Read the model definition and answer for the solid it produces. Units are mm, in the model's axes. Face numbers are marked on the shaded views. A direction names the side the tool comes from. Coordinates: 2 decimals unless noted, no trailing zeros. Loops run counter-clockwise (first coordinate to the right, second up) from the corner with the lowest first, then second, coordinate; pieces in that order, holes last. Notation, with made-up numbers: (-27.5, -12.5) -> (-20.5, -12.5) arc R19 cw to (-20.5, 17.5) -> close; hole circle Ø4 at (47.5, 43.5). An arc over 180 degrees is marked (long way). Answer as CSV lines item,"result".
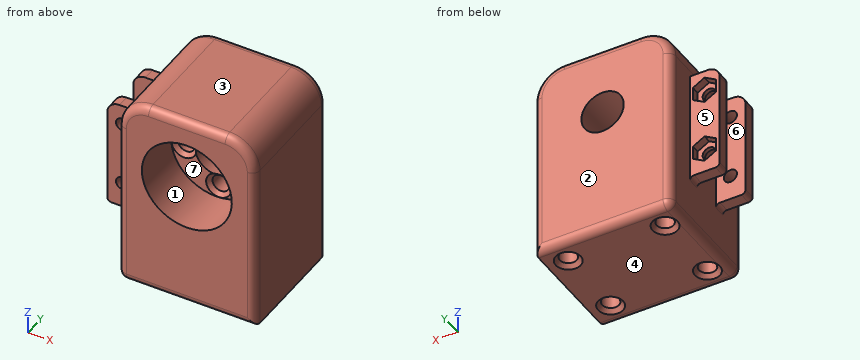
```python
from build123d import *

# Parameters (mm, degrees)
SKETCH1_W           = 34
SKETCH1_H           = 30
BOSS_EXTRUDE1_DEPTH = 49
SKETCH2_R           = 2.1
CUT_EXTRUDE1_DEPTH  = 6
SKETCH5_R           = 11.15
CUT_EXTRUDE2_DEPTH  = 12.5
SKETCH6_R           = 5.25
CUT_EXTRUDE3_DEPTH  = 17.5
SKETCH7_R           = 2.1
CUT_EXTRUDE4_DEPTH  = 6
CHAMFER1_SIZE       = 1
CHAMFER2_SIZE       = 1
FILLET1_R           = 7.5
FILLET2_R           = 2
BOSS_EXTRUDE2_START = 4
SKETCH9_W           = 7.353949633
SKETCH9_H           = 27.286831646
SKETCH9_R           = 1.625
BOSS_EXTRUDE2_DEPTH = 3
FILLET3_R           = 3
FILLET4_R           = 1
CUT_EXTRUDE6_DEPTH  = 2


with BuildPart() as part:
    # Sketch1 → Boss-Extrude1 (new body)
    with BuildSketch(Plane.XY):
        Rectangle(SKETCH1_W, SKETCH1_H)
    extrude(amount=BOSS_EXTRUDE1_DEPTH)

    # Sketch2 → Cut-Extrude1 (cut)
    with BuildSketch(Plane(origin=(0, 0, 0), x_dir=(-1, 0, 0), z_dir=(0, 0, -1))):
        with Locations((12, -9)):
            Circle(SKETCH2_R)
        with Locations((12, 9)):
            Circle(SKETCH2_R)
        with Locations((-12, -9)):
            Circle(SKETCH2_R)
        with Locations((-12, 9)):
            Circle(SKETCH2_R)
    extrude(amount=-CUT_EXTRUDE1_DEPTH, mode=Mode.SUBTRACT)

    # Sketch5 → Cut-Extrude2 (cut)
    with BuildSketch(Plane.XZ.offset(15)):
        with Locations(Location((0, 31.713602896, 0), (0, 0, 270))):
            Circle(SKETCH5_R)
    extrude(amount=-CUT_EXTRUDE2_DEPTH, mode=Mode.SUBTRACT)

    # Sketch6 → Cut-Extrude3 (cut)
    with BuildSketch(Plane(origin=(0, 15, 0), x_dir=(1, 0, 0), z_dir=(0, 1, 0))):
        with Locations(Location((0, -31.713602896, 0), (0, 0, 270))):
            Circle(SKETCH6_R)
    extrude(amount=-CUT_EXTRUDE3_DEPTH, mode=Mode.SUBTRACT)

    # Sketch7 → Cut-Extrude4 (cut)
    with BuildSketch(Plane.XZ.offset(2.5)):
        with Locations(Location((-7.978464084, 31.126993267, 0), (0, 0, 270))):
            Circle(SKETCH7_R)
        with Locations(Location((-0.586609629, 39.692066981, 0), (0, 0, 270))):
            Circle(SKETCH7_R)
        with Locations(Location((7.978464084, 31.126993267, 0), (0, 0, 270))):
            Circle(SKETCH7_R)
        with Locations(Location((0.586609629, 23.735138812, 0), (0, 0, 270))):
            Circle(SKETCH7_R)
    extrude(amount=-CUT_EXTRUDE4_DEPTH, mode=Mode.SUBTRACT)

    # Chamfer1
    # the kernel refuses this chamfer: 1 mm, written as the material it takes off along each edge
    with BuildSketch(Plane(origin=(-7.978464084, -2.5, 31.126993267), x_dir=(0, 0, -1), z_dir=(-1, 0, 0))) as chamfer1_piece_1:
        Polygon((2.1 + CHAMFER1_SIZE, 0), (2.1, -CHAMFER1_SIZE), (2.1, 0), align=None)
    revolve(axis=Axis((-7.978464084, -2.5, 31.126993267), (0, -1, 0)), mode=Mode.SUBTRACT)
    with BuildSketch(Plane(origin=(-0.586609629, -2.5, 39.692066981), x_dir=(0, 0, -1), z_dir=(-1, 0, 0))) as chamfer1_piece_2:
        Polygon((2.1 + CHAMFER1_SIZE, 0), (2.1, -CHAMFER1_SIZE), (2.1, 0), align=None)
    revolve(axis=Axis((-0.586609629, -2.5, 39.692066981), (0, -1, 0)), mode=Mode.SUBTRACT)
    with BuildSketch(Plane(origin=(7.978464084, -2.5, 31.126993267), x_dir=(0, 0, -1), z_dir=(-1, 0, 0))) as chamfer1_piece_3:
        Polygon((2.1 + CHAMFER1_SIZE, 0), (2.1, -CHAMFER1_SIZE), (2.1, 0), align=None)
    revolve(axis=Axis((7.978464084, -2.5, 31.126993267), (0, -1, 0)), mode=Mode.SUBTRACT)
    with BuildSketch(Plane(origin=(0.586609629, -2.5, 23.735138812), x_dir=(0, 0, -1), z_dir=(-1, 0, 0))) as chamfer1_piece_4:
        Polygon((2.1 + CHAMFER1_SIZE, 0), (2.1, -CHAMFER1_SIZE), (2.1, 0), align=None)
    revolve(axis=Axis((0.586609629, -2.5, 23.735138812), (0, -1, 0)), mode=Mode.SUBTRACT)

    # Chamfer2
    chamfer2_edges = [part.edges().sort_by_distance(p)[0] for p in [
        (-9.9, 9, 0),
        (14.1, -9, 0),
        (14.1, 9, 0),
        (-9.9, -9, 0),
    ]]
    chamfer(chamfer2_edges, length=CHAMFER2_SIZE)

    # Fillet1
    fillet1_edges = [part.edges().sort_by_distance(p)[0] for p in [
        (-17, 0, 49),
        (17, 0, 49),
    ]]
    fillet(fillet1_edges, radius=FILLET1_R)

    # Fillet2
    # the kernel refuses this fillet: 2 mm, written as the material it takes off along each edge
    with BuildSketch(Plane(origin=(-15, -13, 2), x_dir=(0, 0, -1), z_dir=(0, -1, 0))) as fillet2_piece_1_section:
        Polygon((0, 0), (FILLET2_R, 0), (FILLET2_R, -FILLET2_R), (0, -FILLET2_R), align=None)
    fillet2_piece_1 = extrude(amount=FILLET2_R, mode=Mode.PRIVATE)
    fillet2_piece_1 = fillet2_piece_1 - Plane(origin=(-15, -13, 2), x_dir=(0.7071067811865475, 0, 0.7071067811865475), z_dir=(0, -1, 0)) * Sphere(FILLET2_R, mode=Mode.PRIVATE)
    add(fillet2_piece_1, mode=Mode.SUBTRACT)
    with BuildSketch(Plane(origin=(-15, 13, 2), x_dir=(0, 0, -1), z_dir=(0, 1, 0))) as fillet2_piece_2_section:
        Polygon((0, 0), (FILLET2_R, 0), (FILLET2_R, FILLET2_R), (0, FILLET2_R), align=None)
    fillet2_piece_2 = extrude(amount=FILLET2_R, mode=Mode.PRIVATE)
    fillet2_piece_2 = fillet2_piece_2 - Plane(origin=(-15, 13, 2), x_dir=(0.7071067811865475, 0, 0.7071067811865475), z_dir=(0, 1, 0)) * Sphere(FILLET2_R, mode=Mode.PRIVATE)
    add(fillet2_piece_2, mode=Mode.SUBTRACT)
    with BuildSketch(Plane(origin=(9.5, 15, 41.5), x_dir=(1, 0, 0), z_dir=(0, 0, -1))) as fillet2_piece_3:
        with BuildLine():
            CenterArc((7.5 - FILLET2_R, FILLET2_R), FILLET2_R, 270, 90)
            Line((7.5 - FILLET2_R, 0), (7.5, 0))
            Line((7.5, 0), (7.5, FILLET2_R))
        make_face()
    revolve(axis=Axis((9.5, 15, 41.5), (0, -1, 0)), revolution_arc=90, mode=Mode.SUBTRACT)
    with BuildSketch(Plane(origin=(17, -15, -5), x_dir=(-1, 0, 0), z_dir=(0, 0, 1)), Plane(origin=(17, 15, -5), x_dir=(0, -1, 0), z_dir=(0, 0, 1))) as fillet2_piece_4:
        with BuildLine():
            CenterArc((FILLET2_R, -FILLET2_R), FILLET2_R, 90, 90)
            Line((0, -FILLET2_R), (0, 0))
            Line((0, 0), (FILLET2_R, 0))
        make_face()
    extrude(amount=46.5, mode=Mode.SUBTRACT)
    with BuildSketch(Plane(origin=(-17, -15, 2), x_dir=(1, 0, 0), z_dir=(0, 0, 1)), Plane(origin=(-17, 15, 2), x_dir=(0, -1, 0), z_dir=(0, 0, 1))) as fillet2_piece_5:
        with BuildLine():
            CenterArc((FILLET2_R, FILLET2_R), FILLET2_R, 180, 90)
            Line((0, FILLET2_R), (0, 0))
            Line((0, 0), (FILLET2_R, 0))
        make_face()
    extrude(amount=39.5, mode=Mode.SUBTRACT)
    with BuildSketch(Plane(origin=(-9.5, -15, 41.5), x_dir=(-1, 0, 0), z_dir=(0, 0, -1))) as fillet2_piece_6:
        with BuildLine():
            CenterArc((7.5 - FILLET2_R, FILLET2_R), FILLET2_R, 270, 90)
            Line((7.5, FILLET2_R), (7.5, 0))
            Line((7.5, 0), (7.5 - FILLET2_R, 0))
        make_face()
    revolve(axis=Axis((-9.5, -15, 41.5), (0, 1, 0)), revolution_arc=90, mode=Mode.SUBTRACT)
    with BuildSketch(Plane(origin=(9.5, -15, 41.5), x_dir=(1, 0, 0), z_dir=(0, 0, -1))) as fillet2_piece_7:
        with BuildLine():
            CenterArc((7.5 - FILLET2_R, -FILLET2_R), FILLET2_R, 0, 90)
            Line((7.5, -FILLET2_R), (7.5, 0))
            Line((7.5, 0), (7.5 - FILLET2_R, 0))
        make_face()
    revolve(axis=Axis((9.5, -15, 41.5), (0, -1, 0)), revolution_arc=90, mode=Mode.SUBTRACT)
    with BuildSketch(Plane(origin=(22, -15, 0), x_dir=(0, 0, 1), z_dir=(-1, 0, 0))) as fillet2_piece_8:
        with BuildLine():
            CenterArc((FILLET2_R, FILLET2_R), FILLET2_R, 180, 90)
            Line((0, FILLET2_R), (0, 0))
            Line((0, 0), (FILLET2_R, 0))
        make_face()
    extrude(amount=37, mode=Mode.SUBTRACT)
    with BuildSketch(Plane(origin=(-17, -13, 0), x_dir=(1, 0, 0), z_dir=(0, 1, 0))) as fillet2_piece_9:
        with BuildLine():
            CenterArc((FILLET2_R, -FILLET2_R), FILLET2_R, 90, 90)
            Line((0, -FILLET2_R), (0, 0))
            Line((0, 0), (FILLET2_R, 0))
        make_face()
    extrude(amount=26, mode=Mode.SUBTRACT)
    with BuildSketch(Plane(origin=(-15, 15, 0), x_dir=(0, -1, 0), z_dir=(1, 0, 0))) as fillet2_piece_10:
        with BuildLine():
            CenterArc((FILLET2_R, -FILLET2_R), FILLET2_R, 90, 90)
            Line((0, -FILLET2_R), (0, 0))
            Line((0, 0), (FILLET2_R, 0))
        make_face()
    extrude(amount=37, mode=Mode.SUBTRACT)
    with BuildSketch(Plane(origin=(-9.5, 15, 49), x_dir=(0, -1, 0), z_dir=(1, 0, 0))) as fillet2_piece_11:
        with BuildLine():
            CenterArc((FILLET2_R, FILLET2_R), FILLET2_R, 180, 90)
            Line((0, FILLET2_R), (0, 0))
            Line((0, 0), (FILLET2_R, 0))
        make_face()
    extrude(amount=19, mode=Mode.SUBTRACT)
    with BuildSketch(Plane(origin=(9.5, -15, 49), x_dir=(0, 0, -1), z_dir=(-1, 0, 0))) as fillet2_piece_12:
        with BuildLine():
            CenterArc((FILLET2_R, -FILLET2_R), FILLET2_R, 90, 90)
            Line((0, -FILLET2_R), (0, 0))
            Line((0, 0), (FILLET2_R, 0))
        make_face()
    extrude(amount=19, mode=Mode.SUBTRACT)
    with BuildSketch(Plane(origin=(-9.5, 15, 41.5), x_dir=(-1, 0, 0), z_dir=(0, 0, -1))) as fillet2_piece_13:
        with BuildLine():
            CenterArc((7.5 - FILLET2_R, -FILLET2_R), FILLET2_R, 0, 90)
            Line((7.5 - FILLET2_R, 0), (7.5, 0))
            Line((7.5, 0), (7.5, -FILLET2_R))
        make_face()
    revolve(axis=Axis((-9.5, 15, 41.5), (0, 1, 0)), revolution_arc=90, mode=Mode.SUBTRACT)

    # Sketch9 → Boss-Extrude2 (add)
    with BuildSketch(Plane(origin=(0, 0, 0), x_dir=(1, 0, 0), z_dir=(0, 1, 0)).offset(BOSS_EXTRUDE2_START)):
        with Locations((-20.676974816, -26.405648135)):
            Rectangle(SKETCH9_W, SKETCH9_H)
        with Locations(Location((-20.6, -35, 0), (0, 0, 270))):
            Circle(SKETCH9_R, mode=Mode.SUBTRACT)
        with Locations(Location((-20.6, -19, 0), (0, 0, 270))):
            Circle(SKETCH9_R, mode=Mode.SUBTRACT)
    boss_extrude2 = extrude(amount=BOSS_EXTRUDE2_DEPTH)

    # Mirror1: Boss-Extrude2 across plane
    add(boss_extrude2.mirror(Plane.ZX))

    # Fillet3
    fillet3_edges = [part.edges().sort_by_distance(p)[0] for p in [
        (-24.353949633, 5.5, 40.049063958),
        (-24.353949633, -5.5, 40.049063958),
    ]]
    fillet(fillet3_edges, radius=FILLET3_R)

    # Fillet4
    fillet4_edges = [part.edges().sort_by_distance(p)[0] for p in [
        (-17, 5.5, 12.762232312),
        (-24.353949633, 5.5, 12.762232312),
        (-17, -5.5, 12.762232312),
        (-24.353949633, -5.5, 12.762232312),
    ]]
    fillet(fillet4_edges, radius=FILLET4_R)

    # Sketch10 → Cut-Extrude6 (cut)
    with BuildSketch(Plane(origin=(0, 7, 0), x_dir=(1, 0, 0), z_dir=(0, 1, 0))):
        Polygon((-17.725, -20.659882024), (-17.725, -17.340117976), (-20.6, -15.680235952), (-23.475, -17.340117976), (-23.475, -20.659882024), (-20.6, -22.319764048), align=None)
        Polygon((-17.725, -36.659882024), (-17.725, -33.340117976), (-20.6, -31.680235952), (-23.475, -33.340117976), (-23.475, -36.659882024), (-20.6, -38.319764048), align=None)
    extrude(amount=-CUT_EXTRUDE6_DEPTH, mode=Mode.SUBTRACT)


solid = part.part
```
Q1. A cutting plane is placed at C-C, the plane y = -9. Write down the section's boundary in (x, z), and give its area (3 significant figures).
Results:
outline,"(-17, 2) arc R2 ccw to (-15.1, 0) -> (-14.1, 1) -> (-14.1, 6) -> (-9.9, 6) -> (-9.9, 1) -> (-8.9, 0) -> (8.9, 0) -> (9.9, 1) -> (9.9, 6) -> (14.1, 6) -> (14.1, 1) -> (15.1, 0) -> (17, 0) -> (17, 41.5) arc R7.5 ccw to (9.5, 49) -> (-9.5, 49) arc R7.5 ccw to (-17, 41.5) -> close; hole circle Ø22.3 at (0, 31.71)"
area,"1,200 mm²"
Q2. For the marked faces 4, 5, 6 and 7, determine the directions among +Z, -Z, +X, -X, +Y, -Y from which every point of the face is accessible in a straight line to the end or side of a thin tool.
Results:
face 4,"-Z, +X, -X, +Y, -Y"
face 5,"+Z, -Z, -X, +Y"
face 6,"+Z, -Z, -X"
face 7,"-Y"
Q3. A cutting plane is placed at A-A, the plane z = 3. Write down the section's boundary in (x, y).
Results:
outline,"(-17, -13) arc R2 ccw to (-15, -15) -> (15, -15) arc R2 ccw to (17, -13) -> (17, 13) arc R2 ccw to (15, 15) -> (-15, 15) arc R2 ccw to (-17, 13) -> close; hole circle Ø4.2 at (-12, -9); hole circle Ø4.2 at (-12, 9); hole circle Ø4.2 at (12, -9); hole circle Ø4.2 at (12, 9)"
Q4. A cutting plane is placed at B-B, the plane z = 19. Write down the section's boundary in (x, y) (3 decimals), and give its area (3 significant figures).
Results:
outline,"(-24.354, -7) -> (-22.225, -7) -> (-22.225, -4) -> (-24.354, -4) -> close; (-24.354, 4) -> (-22.225, 4) -> (-22.225, 5) -> (-23.475, 5) -> (-23.475, 7) -> (-24.354, 7) -> close; (-18.975, -7) -> (-17, -7) -> (-17, -13) arc R2 ccw to (-15, -15) -> (15, -15) arc R2 ccw to (17, -13) -> (17, 13) arc R2 ccw to (15, 15) -> (-15, 15) arc R2 ccw to (-17, 13) -> (-17, 7) -> (-17.725, 7) -> (-17.725, 5) -> (-18.975, 5) -> (-18.975, 4) -> (-17, 4) -> (-17, -4) -> (-18.975, -4) -> close"
area,"1,040 mm²"
Q5. Given pin 1 Ø1.3 at (x, z) = (7.5, 30.5) entering from -Y; pin 2 Ø18 at (x, z) = (0, 31.71) entering from -Y; pin 3 Ø6.5 at (x, z) = (-20.5, 35.5) entering from +Y, each flat-ended and moving along its own axis, determine where each tip first touches the part or whether it passes through.
Results:
pin 1,"stops at y = 3.5"
pin 2,"stops at y = -2.5"
pin 3,"stops at y = 7"
Q6. Find the intervals of material crossed by probe 1 along Y at (x, z) = (12, 4.15); probe 2 along X at (y, z) = (-5.5, 32); probe 3 along Z at (x, y) = (0, 7.75), in increasing order. Write a range as [from, to].
Results:
probe 1,"y = [-15, -11.1], [-6.9, 6.9], [11.1, 15]"
probe 2,"x = [-24.35, -11.15], [11.15, 17]"
probe 3,"z = [0, 26.46], [36.96, 49]"
Q7. For a pull along Z with two mould halves and no side action, classify the marked faces 1, 2 and 3 as pulls with the +Z half, pulls with the -Z half, needs draft (parallel to the pull), parting line crosses it, or undercut.
Results:
face 1,"undercut"
face 2,"needs draft"
face 3,"pulls with the +Z half"
Q8. A cutting plane is placed at D-D, the plane y = 9. Write down the section's boundary in (x, z), and give its area (3 significant figures).
Results:
outline,"(-17, 2) arc R2 ccw to (-15.1, 0) -> (-14.1, 1) -> (-14.1, 6) -> (-9.9, 6) -> (-9.9, 1) -> (-8.9, 0) -> (8.9, 0) -> (9.9, 1) -> (9.9, 6) -> (14.1, 6) -> (14.1, 1) -> (15.1, 0) -> (17, 0) -> (17, 41.5) arc R7.5 ccw to (9.5, 49) -> (-9.5, 49) arc R7.5 ccw to (-17, 41.5) -> close; hole circle Ø10.5 at (0, 31.71)"
area,"1,500 mm²"
